Study the drawing (mm; zero at the part's minimum x, y, z) and answer. A direction names the side the tool comes from. Round coordinates to 2 decimals unless told otherwise and drop trailing zeros. Order: outer loops, then holes, each group sorted by start corner. A loop starts at its lowest first (then second) coordinate and runs counter-clockwise, first axis right, second up. Notation, with made-up numbers: (-36, 21) - (-28, 21) arc R13 cw to (-28, 40) - close; hole circle Ø11 at (88.25, 39). An arc over 180 degrees is marked (long way). Put each result on its own line as item: value.
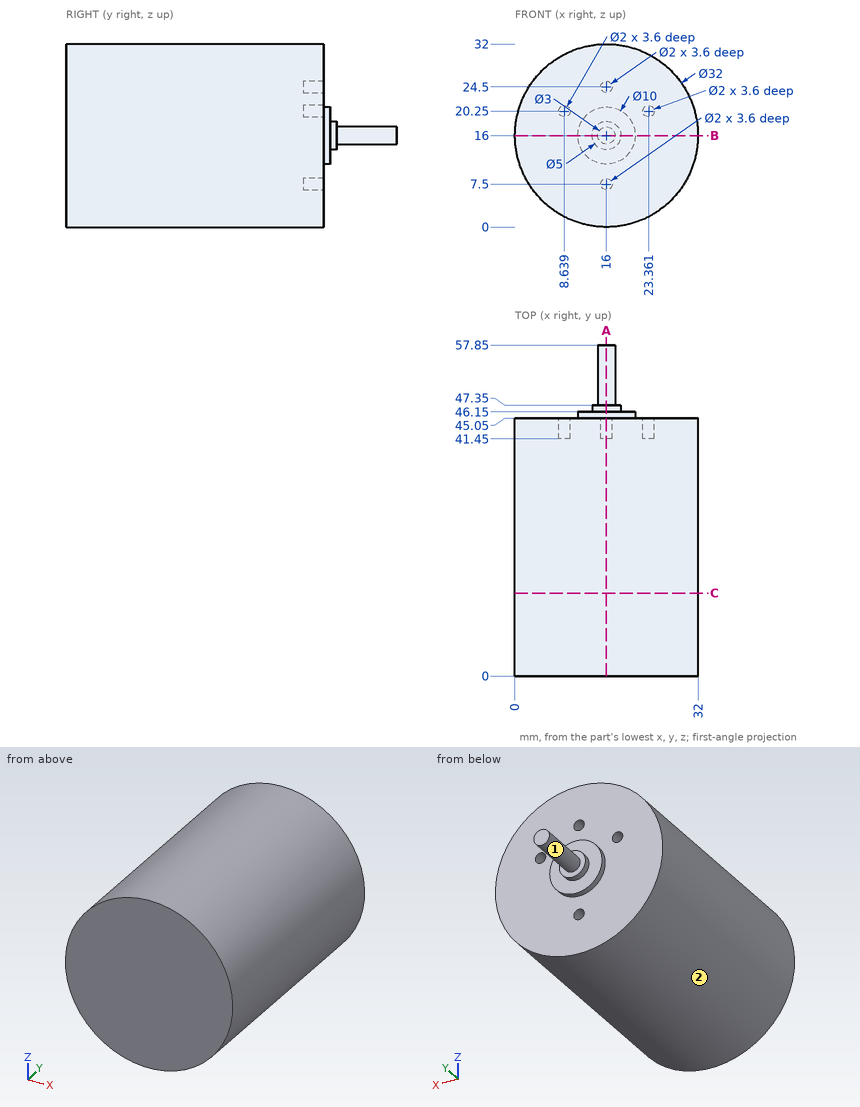
1) A cutting plane is placed at C-C on y = 14.5. Write down the section's boundary in (x, z).
Findings below:
outline: circle Ø32 at (16, 16)
2) A cutting plane is placed at B-B on z = 16. Write down the section's boundary in (x, y).
Findings below:
outline: (0, 0) - (32, 0) - (32, 45.05) - (21, 45.05) - (21, 46.15) - (18.5, 46.15) - (18.5, 47.35) - (17.5, 47.35) - (17.5, 57.85) - (14.5, 57.85) - (14.5, 47.35) - (13.5, 47.35) - (13.5, 46.15) - (11, 46.15) - (11, 45.05) - (0, 45.05) - close
3) For the marked faces 1 and 2, determine the directions among +Z, -Z, +X, -X, +Y, -Y from which every point of the face is accessible in a straight line to the end or side of a thin tool.
Findings below:
face 1: +Y
face 2: +Y, -Y
4) Straight lines are drawn through the part: L1, parallel to X at y = 43, z = 20; L2, parallel to Y at x = 23, z = 16; L3, parallel to X at y = 42.7, z = 20.25 (1 decimal). For each, find the intervals that lie inside material, in ascending order. Write a range as from..to.
Findings below:
L1: x = 0.51..7.67, 9.61..22.39, 24.33..31.49
L2: y = 0..45.05
L3: x = 0.6..7.6, 9.6..22.4, 24.4..31.4
5) A cutting plane is placed at A-A on x = 16. Write down the section's boundary in (y, z).
Findings below:
outline: (0, 0) - (45.05, 0) - (45.05, 6.5) - (41.45, 6.5) - (41.45, 8.5) - (45.05, 8.5) - (45.05, 11) - (46.15, 11) - (46.15, 13.5) - (47.35, 13.5) - (47.35, 14.5) - (57.85, 14.5) - (57.85, 17.5) - (47.35, 17.5) - (47.35, 18.5) - (46.15, 18.5) - (46.15, 21) - (45.05, 21) - (45.05, 23.5) - (41.45, 23.5) - (41.45, 25.5) - (45.05, 25.5) - (45.05, 32) - (0, 32) - close
6) Given pin 1 Ø2.5 at (x, z) = (16, 24.5) entering from +Y; pin 2 Ø4 at (x, y) = (27, 26) entering from +Z; pin 3 Ø12 at (y, z) = (42.5, 23.5) entering from +X, each flat-ended and moving along its own axis, determine where each tip first touches the part or whether it passes through.
Findings below:
pin 1: stops at y = 45.05
pin 2: stops at z = 29.23
pin 3: stops at x = 31.93
